Could you check a few things on this model? Use its own coordinates, in mm. Face numbers are marked on the shaded views. Round coordinates to 2 decimals unless told otherwise and drop trailing zeros. Order: outer loops, then holes, each group sorted by start corner. A loop starts at its lowest first (then second) coordinate and runs counter-clockwise, first axis right, second up. Notation, with made-up numbers: (-33.75, -16) -> (13.25, -16) arc R6 cw to (13.25, -10) -> close; hole circle Ø10 at (75.5, 58). An arc over 180 degrees is marked (long way). Put each result on its own line as item: value. Start each with the question number.
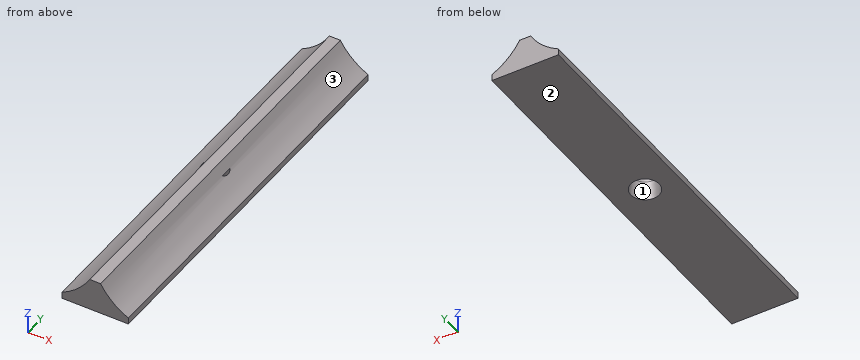
from build123d import *

# Parameters (mm, degrees)
BOSS_EXTRUDE1_DEPTH = 30


with BuildPart() as part:
    # Sketch1 → Boss-Extrude1 (new, symmetric)
    with BuildSketch(Plane(origin=(0, 0, 0), x_dir=(1, 0, 0), z_dir=(0, 1, 0))):
        with BuildLine():
            Line((-0.839745962, 0), (0.839745962, 0))
            ThreePointArc((0.839745962, 0), (2.690111154, 2.322937519), (5.141101056, 4))
            Line((5.141101056, 4), (5.141101056, 5))
            Line((5.141101056, 5), (-5.141101056, 5))
            Line((-5.141101056, 5), (-5.141101056, 4))
            ThreePointArc((-5.141101056, 4), (-2.690111154, 2.322937519), (-0.839745962, 0))
        make_face()
    extrude(amount=BOSS_EXTRUDE1_DEPTH, both=True)

    # Sketch8 → #24 (0.152) Diameter Hole1 (revolve, cut)
    with BuildSketch(Plane(origin=(0, 0, -5), x_dir=(0, 1, 0), z_dir=(1, 0, 0))):
        Polygon((0, 0), (0, 3.7), (1.999999937, 3.7), (1.999999937, 2.860134796), (2.200000045, 0), align=None)
    revolve(axis=Axis((0, 0, -11.35), (0, 0, 1)), mode=Mode.SUBTRACT)


solid = part.part
1. If we section it at C-C, the plane z = -3.4: Please give me the cut outline in (x, y), then the cut area to 3 significant figures.
2. If we section it at A-A, the plane x = 0: Please give me the cut outline in (y, z), then the cut area to 3 significant figures.
3. If we section it at D-D, the plane y = 18: Please give me the cut outline in (x, z).
4. Thinking about a two-plate mould opening in X: for the marked faces 1, 2 and 3, which applies, +X half, -X half, draft (parallel to the pull), parting line (faces both ways), or undercut?
5. For pin 1 Ø1 at (x, y) = (2.5, 6) entering from +Z; pin 2 Ø1 at (x, y) = (0, -0.5) entering from -Z, each with a flat end and sliding along its axis, tell me the tip position at first contact or that it passes through.
6. I need wall thicknesses on L1, parallel to Y at x = 0, z = -1.9; L2, parallel to Y at x = -0.5, z = -4.7; L3, parallel to Z at x = -4, y = 1. Which ranges of each line are inside material? Lowest first, please.
7. If we section it at B-B, the plane y = 0: Please give me the cut outline in (x, z).
Results below:
1. outline: (-4.07, -30) -> (4.07, -30) -> (4.07, 30) -> (-4.07, 30) -> close; hole circle Ø4.18 at (0, 0)
1. area: 475 mm2
2. outline: (-30, -5) -> (-2.2, -5) -> (-2, -2.14) -> (-2, -1.3) -> (2, -1.3) -> (2, -2.14) -> (2.2, -5) -> (30, -5) -> (30, 0) -> (-30, 0) -> close
2. area: 285 mm2
3. outline: (-5.14, -5) -> (5.14, -5) -> (5.14, -4) arc R10 cw to (0.84, 0) -> (-0.84, 0) arc R10 cw to (-5.14, -4) -> close
4. face 1: undercut
4. face 2: draft
4. face 3: +X half
5. pin 1: z = -1.61
5. pin 2: z = -1.3
6. L1: -30 to -2, 2 to 30
6. L2: -30 to -2.12, 2.12 to 30
6. L3: -5 to -3.35
7. outline: (-5.14, -5) -> (-2.2, -5) -> (-2, -2.14) -> (-2, -1.61) arc R10 cw to (-5.14, -4) -> close; (-1.73, -1.3) -> (1.73, -1.3) arc R10 cw to (0.84, 0) -> (-0.84, 0) arc R10 cw to start; (2, -2.14) -> (2.2, -5) -> (5.14, -5) -> (5.14, -4) arc R10 cw to (2, -1.61) -> close
